Geometry check sheet. Reference: the model listing, model coordinates, mm. Face numbers are marked on the shaded views. A direction names the side the tool comes from. Give positions to 0.01 mm unless a question says otherwise; leave off trailing zeros. Order: outer loops, then holes, each group sorted by start corner. A loop starts at its lowest first (then second) coordinate and runs counter-clockwise, first axis right, second up.
from build123d import *

# Parameters (mm, degrees)
SKETCH1_W           = 44.45
SKETCH1_H           = 88.9
BOSS_EXTRUDE1_DEPTH = 76.2
CUT_EXTRUDE1_DEPTH  = 76.2
SKETCH3_W           = 25.4
SKETCH3_H           = 6.35
BOSS_EXTRUDE2_DEPTH = 31.75
FILLET1_R           = 2.54
SKETCH4_R           = 6.477
CUT_EXTRUDE2_DEPTH  = 38.1
SKETCH5_W           = 25.4
SKETCH5_H           = 6.35
BOSS_EXTRUDE3_DEPTH = 31.75
FILLET2_R           = 2.54


with BuildPart() as part:
    # Sketch1 → Boss-Extrude1 (new body)
    with BuildSketch(Plane(origin=(0, 0, 0), x_dir=(1, 0, 0), z_dir=(0, 1, 0))):
        with Locations((22.225, 44.45)):
            Rectangle(SKETCH1_W, SKETCH1_H)
    extrude(amount=BOSS_EXTRUDE1_DEPTH)

    # Sketch2 → Cut-Extrude1 (cut)
    with BuildSketch(Plane(origin=(44.45, 0, 0), x_dir=(0, 0, -1), z_dir=(1, 0, 0))):
        Polygon((44.45, 23.226552809), (44.45, 0), (88.9, 0), (88.9, 76.2), (0, 76.2), align=None)
    extrude(amount=-CUT_EXTRUDE1_DEPTH, mode=Mode.SUBTRACT)

    # Sketch3 → Boss-Extrude2 (add)
    with BuildSketch(Plane(origin=(44.45, 0, 0), x_dir=(0, 0, -1), z_dir=(1, 0, 0))):
        with Locations((12.7, 3.175)):
            Rectangle(SKETCH3_W, SKETCH3_H)
    extrude(amount=BOSS_EXTRUDE2_DEPTH)

    # Fillet1
    fillet1_edges = [part.edges().sort_by_distance(p)[0] for p in [
        (44.45, 6.35, -12.7),
    ]]
    fillet(fillet1_edges, radius=FILLET1_R)

    # Sketch4 → Cut-Extrude2 (cut)
    with BuildSketch(Plane(origin=(0, 6.35, 0), x_dir=(1, 0, 0), z_dir=(0, 1, 0))):
        with Locations(Location((61.595, 12.7, 0), (0, 0, 270))):
            Circle(SKETCH4_R)
    cut_extrude2 = extrude(amount=-CUT_EXTRUDE2_DEPTH, mode=Mode.SUBTRACT)

    # Sketch5 → Boss-Extrude3 (add)
    with BuildSketch(Plane.ZY):
        with Locations((-12.7, 3.175)):
            Rectangle(SKETCH5_W, SKETCH5_H)
    extrude(amount=BOSS_EXTRUDE3_DEPTH)

    # Mirror4: Cut-Extrude2 across plane
    add(cut_extrude2.mirror(Plane(origin=(22.225, 0, 0), x_dir=(0, 0, 1), z_dir=(1, 0, 0))), mode=Mode.SUBTRACT)

    # Fillet2
    fillet2_edges = [part.edges().sort_by_distance(p)[0] for p in [
        (0, 6.35, -12.7),
    ]]
    fillet(fillet2_edges, radius=FILLET2_R)


solid = part.part
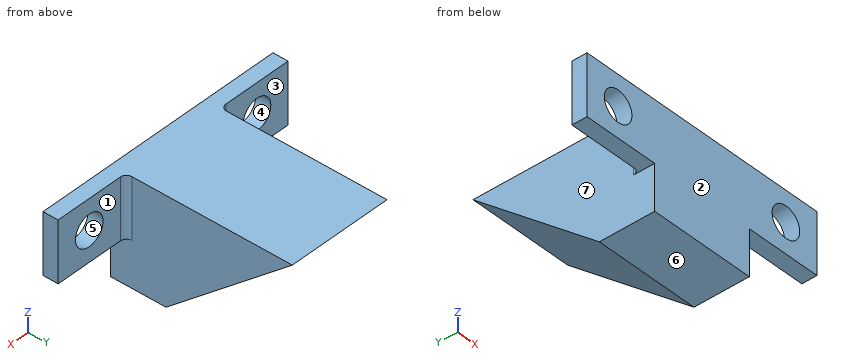
Item 1: Sectioned sample at B-B (z = -22.5). Enter the section's corners in (x, y).
Reported:
outline: (-31.75, 0) - (76.2, 0) - (76.2, 6.35) - (46.99, 6.35) arc R2.54 cw to (44.45, 8.89) - (44.45, 49.39) - (0, 49.39) - (0, 8.89) arc R2.54 cw to (-2.54, 6.35) - (-31.75, 6.35) - close
Item 2: Sectioned sample at C-C (y = 58.5). Enter the section's corners in (x, z).
Reported:
outline: (0, -14.85) - (44.45, -14.85) - (44.45, 0) - (0, 0) - close
Item 3: Draft check along Z on the marked faces 4, 5, 6 and 7. Enter one of: released by +Z, released by -Z, zero draft, split by the parting line, or undercut.
Reported:
face 4: undercut
face 5: undercut
face 6: released by -Z
face 7: zero draft
Item 4: Sectioned sample at D-D (y = 68). Enter the section's corners in (x, z), and give its area (3 significant figures).
Reported:
outline: (0, -6.88) - (44.45, -6.88) - (44.45, 0) - (0, 0) - close
area: 306 mm2
Item 5: Gauge pin test, flat ends, axial feed: pin 1 (4 mm diameter, centred on x = 23, y = 30, fed in from -Z); pin 2 (13.5 mm diameter, centred on y = 38.5, z = -23.5, fed in from -X); pin 3 (22 mm diameter, centred on y = 53.5, z = -16.5, fed in from +X). Record the tip position at first contact, or that the pin passes through.
Reported:
pin 1: stops at z = -40.44
pin 2: stops at x = 0
pin 3: stops at x = 44.45
Item 6: Sectioned sample at A-A (z = -12.7). Enter the section's corners in (x, y), and give its area (3 significant figures).
Reported:
outline: (-31.75, 0) - (-23.62, 0) - (-23.62, 6.35) - (-31.75, 6.35) - close; (-10.67, 0) - (55.12, 0) - (55.12, 6.35) - (46.99, 6.35) arc R2.54 cw to (44.45, 8.89) - (44.45, 61.06) - (0, 61.06) - (0, 8.89) arc R2.54 cw to (-2.54, 6.35) - (-10.67, 6.35) - close; (68.07, 0) - (76.2, 0) - (76.2, 6.35) - (68.07, 6.35) - close
area: 2,960 mm2
Item 7: Set-up check for the marked faces 1, 2 and 3: record each of +Z, -Z, +X, -X, +Y, -Y from which the full face is reachable in a straight line by a thin tool's end or side.
Reported:
face 1: +Z, -Z, +X, +Y
face 2: +Z, -Z, +X, -X, -Y
face 3: +Z, -Z, -X, +Y
Item 8: Scan lines: L1, parallel to X at y = 2, z = -12.7; L2, parallel to X at y = 2, z = -12; L3, parallel to X at y = 34.5, z = -5.5. Record each from-to range of solid material in increasing order.
Reported:
L1: x = -31.75 to -23.62, -10.67 to 55.12, 68.07 to 76.2
L2: x = -31.75 to -23.58, -10.71 to 55.16, 68.03 to 76.2
L3: x = 0 to 44.45
